from build123d import *

# Parameters (mm, degrees)
PAD_DEPTH    = 5
PAD001_DEPTH = 3.2
PAD002_DEPTH = 5
POCKET_DEPTH = 3.2
PAD003_DEPTH = 16.8
PAD004_DEPTH = 16.8
SKETCH006_W  = 10
SKETCH006_H  = 10
PAD005_DEPTH = 20


with BuildPart() as part:
    # Sketch → Pad (new body)
    with BuildSketch(Plane.XY):
        Polygon((0, 0), (70, 0), (70, 30), (30, 30), (30, 70), (0, 70), align=None)
    extrude(amount=PAD_DEPTH)

    # Sketch001 (on DatumPlane) → Pad001 (join)
    with BuildSketch(Plane.XY.offset(5)):
        Polygon((0, 0), (70, 0), (70, 10), (10, 10), (10, 70), (0, 70), align=None)
    extrude(amount=PAD001_DEPTH)

    # Sketch002 (on DatumPlane) → Pad002 (join)
    with BuildSketch(Plane.XY.offset(8.2)):
        Polygon((0, 0), (70, 0), (70, 30), (30, 30), (30, 70), (0, 70), align=None)
    extrude(amount=PAD002_DEPTH)

    # Sketch003 (on DatumPlane) → Pocket (cut)
    with BuildSketch(Plane.XY.offset(13.2)):
        Polygon((5, 70), (5, 5), (70, 5), (70, 8.2), (8.2, 8.2), (8.2, 70), align=None)
    extrude(amount=-POCKET_DEPTH, mode=Mode.SUBTRACT)

    # Sketch004 (on DatumPlane) → Pad003 (join)
    with BuildSketch(Plane.XY.offset(13.2)):
        Polygon((0, 0), (0, 70), (5, 70), (5, 5), (70, 5), (70, 0), align=None)
    extrude(amount=PAD003_DEPTH)

    # Sketch005 (on DatumPlane) → Pad004 (join)
    with BuildSketch(Plane.XY.offset(13.2)):
        Polygon((70, 8.2), (70, 13.2), (13.2, 13.2), (13.2, 70), (8.2, 70), (8.2, 8.2), align=None)
    extrude(amount=PAD004_DEPTH)

    # Sketch006 (on DatumPlane) → Pad005 (join)
    with BuildSketch(Plane.XY.offset(10)):
        with Locations((5, 5)):
            Rectangle(SKETCH006_W, SKETCH006_H)
    extrude(amount=PAD005_DEPTH)


solid = part.part
Geometry check sheet. Reference: the model listing, model coordinates, mm. A direction names the side the tool comes from. Give positions to 0.01 mm unless a question says otherwise; leave off trailing zeros. Loops run counter-clockwise (first coordinate to the right, second up) from the corner with the lowest first, then second, coordinate; pieces in that order, holes last. Notation, with made-up numbers: M 70.25,57.25 L 81.25,57.25 A20 cw 81.25,88.25 Z; hole C -1,65.5 d9. An arc over 180 degrees is marked long. Write each question's results on one line, items separated by ' | '.
1) Release check for a two-part mould opening along X. For faces 5 (the face through (50, 30, 11)), 6 (the face through (30, 50, 2)), 7 (the face through (8.2, 40, 20)), 8 (the face through (0, 35, 15)) record: +X half, -X half, draft (parallel to the pull), parting line (faces both ways), or undercut.
Answers follow:
face 5: draft | face 6: +X half | face 7: undercut | face 8: -X half
2) Thickness scan on line 1 (X direction, y = 66, z = 18); line 2 (Y direction, x = 44.5, z = 10.5). Record the ranges inside material, lowest first.
Answers follow:
line 1: 0 to 5, 8.2 to 13.2 | line 2: 0 to 5, 8.2 to 30
3) Section check A-A, the plane x = 59. Record the boundary of the cut face in (y, z), plus the area to 3 significant figures.
Answers follow:
outline: M 0,0 L 30,0 L 30,5 L 10,5 L 10,8.2 L 30,8.2 L 30,13.2 L 13.2,13.2 L 13.2,30 L 8.2,30 L 8.2,10 L 5,10 L 5,30 L 0,30 Z | area: 490 mm2
4) Section check C-C, the plane z = 3.5. Record the boundary of the cut face in (x, y), plus the area to 3 significant figures.
Answers follow:
outline: M 0,0 L 70,0 L 70,30 L 30,30 L 30,70 L 0,70 Z | area: 3,300 mm2
5) Gauge pin test, flat ends, axial feed: pin 1 (6 mm diameter, centred on y = 19.5, z = 23.5, fed in from +X); pin 2 (10 mm diameter, centred on x = 42.5, y = 32.5, fed in from +Z); pin 3 (1 mm diameter, centred on x = 27, y = 7, fed in from +Z); pin 4 (17 mm diameter, centred on x = 43.5, y = 39.5, fed in from +Z). Record the tip position at first contact, or that the pin passes through.
Answers follow:
pin 1: x = 13.2 | pin 2: z = 13.2 | pin 3: z = 10 | pin 4: through
6) Section check B-B, the plane z = 17.75. Record the boundary of the cut face in (x, y).
Answers follow:
outline: M 0,0 L 70,0 L 70,5 L 10,5 L 10,8.2 L 70,8.2 L 70,13.2 L 13.2,13.2 L 13.2,70 L 8.2,70 L 8.2,10 L 5,10 L 5,70 L 0,70 Z
7) Tool access check on faces 1 (the face through (29, 36, 13.2)), 2 (the face through (40, 10, 7)), 3 (the face through (7, 40, 10)), 4 (the face through (40, 5, 20)). Record the directions out of +Z, -Z, +X, -X, +Y, -Y that give a thin tool (end or side, any length) a straight path to the whole face; none if there is none.
Answers follow:
face 1: +Z, +X, +Y | face 2: +X, +Y | face 3: +Z, +Y | face 4: +Z, +X
